Geometry: final body of the model. Coordinates: model frame, mm. A direction names the side the tool comes from. Give positions to 0.01 mm unless a question says otherwise; leave off trailing zeros. Loops run counter-clockwise (first coordinate to the right, second up) from the corner with the lowest first, then second, coordinate; pieces in that order, holes last. Notation, with made-up numbers: (63, 77.5) - (109, 77.5) arc R30 cw to (109, 100.5) - close; hole circle Ø5 at (-5.75, -15). An arc over 180 degrees is marked (long way). Use one line per item in the form item = value.
Autodesk Fusion 360 part; units mm, degrees
sketch "Sketch2" plane through (0, 0, 0) normal (0, 0, 1) x (1, 0, 0)
  line L0 (0, 0) -> (147.5, 0)
  line L1 (147.5, 0) -> (147.5, 58.5)
  line L2 (147.5, 58.5) -> (0, 58.5)
  line L3 (0, 58.5) -> (0, 0)
  line L4 (69.75, 0) -> (77.75, 0)
  line L5 (77.75, 0) -> (77.75, -8)
  line L6 (77.75, -8) -> (69.75, -8)
  line L7 (69.75, -8) -> (69.75, 0)
  line L8 (147.5, 24.75) -> (147.5, 32.75)
  line L9 (147.5, 32.75) -> (155.5, 32.75)
  line L10 (155.5, 32.75) -> (155.5, 24.75)
  line L11 (155.5, 24.75) -> (147.5, 24.75)
  line L12 (73.75, 58.5) -> (73.75, 0) construction
  line L13 (147.5, 28.75) -> (155.5, 28.75) construction
  line L14 (151.5, 32.75) -> (151.5, 24.75) construction
  circle A0 centre (151.5, 28.75) radius 1.875
  line L15 (-8, 24.75) -> (0, 24.75)
  line L16 (-8, 32.75) -> (-8, 24.75)
  line L17 (0, 32.75) -> (-8, 32.75)
  circle A1 centre (-4, 28.75) radius 1.875
  line L18 (69.75, -4) -> (77.75, -4) construction
  line L19 (73.75, 0) -> (73.75, -8) construction
  circle A2 centre (73.75, -4) radius 1.875
  point P0 (73.75, 0)
  point P1 (147.5, 28.75)
  point P2 (-8, 28.75)
  dimension "d8" = 147.5
  dimension "d9" = 58.5
  dimension "d12" = 8
  dimension "d13" = 8
  dimension "d14" = 8
  dimension "d15" = 8
  dimension "d16" = 8
  dimension "d17" = 3.75
  dimension "d18" = 3.75
extrude "Extrude1" add sketch "Sketch2" along normal blind 3
fillet "Fillet1" radius 1.5 12 edges at (77.75, 0, 1.5) (77.75, -8, 1.5) (69.75, -8, 1.5) (69.75, 0, 1.5) (0, 24.75, 1.5) (-8, 24.75, 1.5) (-8, 32.75, 1.5) (0, 32.75, 1.5) (155.5, 32.75, 1.5) (147.5, 32.75, 1.5) (147.5, 24.75, 1.5) (155.5, 24.75, 1.5)
sketch "Sketch3" plane through (0, 0, 3) normal (0, 0, 1) x (-1, 0, 0)
  arc A0 (-154, -24.75) -> (-155.5, -26.25) centre (-154, -26.25) ccw
  line L0 (-155.5, -26.25) -> (-155.5, -31.25)
  arc A1 (-155.5, -31.25) -> (-154, -32.75) centre (-154, -31.25) ccw
  line L1 (-154, -32.75) -> (-149, -32.75)
  arc A2 (-147.5, -34.25) -> (-149, -32.75) centre (-149, -34.25) ccw
  line L2 (-147.5, -34.25) -> (-147.5, -58.5)
  line L3 (-147.5, -58.5) -> (0, -58.5)
  line L4 (0, -58.5) -> (0, -34.25)
  arc A3 (1.5, -32.75) -> (0, -34.25) centre (1.5, -34.25) ccw
  line L5 (1.5, -32.75) -> (6.5, -32.75)
  arc A4 (6.5, -32.75) -> (8, -31.25) centre (6.5, -31.25) ccw
  line L6 (8, -31.25) -> (8, -26.25)
  arc A5 (8, -26.25) -> (6.5, -24.75) centre (6.5, -26.25) ccw
  line L7 (6.5, -24.75) -> (1.5, -24.75)
  arc A6 (0, -23.25) -> (1.5, -24.75) centre (1.5, -23.25) ccw
  line L8 (0, -23.25) -> (0, 0)
  line L9 (0, 0) -> (-68.25, 0)
  arc A7 (-69.75, 1.5) -> (-68.25, 0) centre (-68.25, 1.5) ccw
  line L10 (-69.75, 1.5) -> (-69.75, 6.5)
  arc A8 (-69.75, 6.5) -> (-71.25, 8) centre (-71.25, 6.5) ccw
  line L11 (-71.25, 8) -> (-76.25, 8)
  arc A9 (-76.25, 8) -> (-77.75, 6.5) centre (-76.25, 6.5) ccw
  line L12 (-77.75, 6.5) -> (-77.75, 1.5)
  arc A10 (-79.25, 0) -> (-77.75, 1.5) centre (-79.25, 1.5) ccw
  line L13 (-79.25, 0) -> (-147.5, 0)
  line L14 (-147.5, 0) -> (-147.5, -23.25)
  arc A11 (-149, -24.75) -> (-147.5, -23.25) centre (-149, -23.25) ccw
  line L15 (-149, -24.75) -> (-154, -24.75)
  circle A12 centre (-151.5, -28.75) radius 1.875
  circle A13 centre (4, -28.75) radius 1.875
  circle A14 centre (-73.75, 4) radius 1.875
  line L16 (0, -2.5) -> (-147.5, -2.5) construction
  line L17 (-54.6806, -2.5) -> (-92.6806, -2.5)
  line L18 (-92.6806, -2.5) -> (-92.6806, 0)
  line L19 (-54.6806, -2.5) -> (-54.6806, 0)
  line L20 (-54.6806, 0) -> (-92.6806, 0)
  line L21 (-145, -57) -> (-145, 0) construction
  line L22 (-145, -13.4089) -> (-145, -43.4089)
  line L23 (-145, -43.4089) -> (-147.5, -43.4089)
  line L24 (-145, -13.4089) -> (-147.5, -13.4089)
  line L25 (-147.5, -13.4089) -> (-147.5, -43.4089)
  line L26 (-73.75, -58.5) -> (-73.6806, 0) construction
  line L27 (-2.3933, -13.578) -> (0.1067, -13.5839)
  line L28 (0.1067, -13.5839) -> (0.0356, -43.5838)
  line L29 (-2.4644, -43.5779) -> (0.0356, -43.5838)
  line L30 (-2.3933, -13.578) -> (-2.4644, -43.5779)
  line L31 (0, -56) -> (-147.5, -56) construction
  line L32 (-50.7607, -56.0267) -> (-95.7606, -55.9733)
  line L33 (-95.7606, -55.9733) -> (-95.7606, -58.5)
  line L34 (-50.7607, -56.0267) -> (-50.7607, -58.5)
  line L35 (-50.7607, -58.5) -> (-95.7606, -58.5)
  line L36 (-70.7606, -56.003) -> (-75.7606, -55.997)
  line L37 (-75.7606, -55.997) -> (-75.7611, -58.5)
  line L38 (-75.7611, -58.5) -> (-70.7611, -58.5)
  line L39 (-70.7611, -58.5) -> (-70.7606, -56.003)
  point P0 (-73.6806, -2.5)
  point P1 (-145, -28.4089)
  point P2 (-73.2606, -56)
  point P3 (-73.2606, -56)
  dimension "d23" = 2.5
  dimension "d24" = 38
  dimension "d25" = 2.5
  dimension "d26" = 30
  dimension "d27" = 2.5
  dimension "d28" = 45
  dimension "d29" = 5
extrude "Extrude2" add sketch "Sketch3" along normal blind 15 contours L2 L14 L22 L23 L24 L25 | L9 L13 L17 L18 L19 L20 | L3 L32 L33 L35 L37 | L3 L32 L34 L35 L39 | A6 L8 L27 L28 | L4 A3 A6 L8 L27 L28 L29 L30 | L4 A3 L28 L29
equation "controller_length = 144 mm"
equation "controller_width = 55 mm"
equation "mount_hole_diameter = 3.5 mm"
equation "base_thickness = 3 mm"
equation "wall_thickness = 2.5 mm"
equation "give = 1 mm"
equation "d8 = total_length"
equation "d9 = total_width"
equation "total_length = controller_length + wall_thickness + give"
equation "total_width = controller_width + give + wall_thickness"
equation "d19 = base_thickness"
equation "d23 = wall_thickness"
equation "d25 = wall_thickness"
equation "d27 = wall_thickness"
equation "d30 = wall_height"
equation "wall_height = 15 mm"
(1) Cut plane B-B (y = -4). Return the cut outline in (x, z) (3 decimals), plus the area to 4 significant figures.
Solution:
outline = (69.75, 0) - (71.875, 0) - (71.875, 3) - (69.75, 3) - close; (75.625, 0) - (77.75, 0) - (77.75, 3) - (75.625, 3) - close
area = 12.75 mm2
(2) Access query for faces 1 (the face through (149.7, 27.6, 3)), 2 (the face through (151, 32.75, 1)), 3 (the face through (73, 2.5, 10)). Directions: +Z, -Z, +X, -X, +Y, -Y. A direction counts if a zero-diameter tool reaches every point of the face in a straight line with its end or side. Return the directions, or none.
Solution:
face_1 = +Z, +X, +Y, -Y
face_2 = +Z, -Z, +X, +Y
face_3 = +Z, +X, -X
(3) Cut plane A-A (z = 16). Return the cut outline in (x, y), plus the area to 3 significant figures.
Solution:
outline = (-0.11, 13.58) - (2.39, 13.58) - (2.46, 43.58) - (-0.04, 43.58) - close; (50.76, 56.03) - (70.76, 56) - (70.76, 58.5) - (50.76, 58.5) - close; (54.68, 0) - (92.68, 0) - (92.68, 2.5) - (54.68, 2.5) - close; (75.76, 56) - (95.76, 55.97) - (95.76, 58.5) - (75.76, 58.5) - close; (145, 13.41) - (147.5, 13.41) - (147.5, 43.41) - (145, 43.41) - close
area = 345 mm2
(4) Pull-direction query (Y, two-part tool) for faces 4 (the face through (-4.41, 30.58, 1.48)), 5 (the face through (0, 12, 1)), 6 (the face through (73, 0, 7)), 7 (the face through (72.4, -5.3, 1.5)); classes: released by +Y, released by -Y, zero draft, split by the parting line, or undercut.
Solution:
face_4 = undercut
face_5 = zero draft
face_6 = released by -Y
face_7 = undercut
(5) Cut plane D-D (x = 73.75). Return the cut outline in (y, z) (3 decimals).
Solution:
outline = (-8, 0) - (-5.875, 0) - (-5.875, 3) - (-8, 3) - close; (-2.125, 0) - (58.5, 0) - (58.5, 3) - (2.5, 3) - (2.5, 18) - (0, 18) - (0, 3) - (-2.125, 3) - close
(6) Material intervals for L1, parallel to X at y = 37, z = 16.75; L2, parallel to Y at x = 87, z = 16.75; L3, parallel to Y at x = 73.75, z = 0.9 (3 decimals), sorted ascending. Write a range as from..to.
Solution:
L1 = -0.05..2.45, 145..147.5
L2 = 0..2.5, 55.98..58.5
L3 = -8..-5.875, -2.125..58.5
(7) Pin query (flat end, axial travel): P1, Ø1.5, axis at y = -3.5, z = 1, coming from the +X side; P2, Ø0.9, axis at y = 51.5, z = 2, coming from the -X side; P3, Ø4, axis at x = 74.5, y = -5.5, coming from the +Z side; P4, Ø3.5, axis at x = 73.75, y = -4, coming from the -Z side. Return the tip coordinate at first contact, or that it passes through.
Solution:
P1 = 77.75
P2 = 0
P3 = 3
P4 = through
(8) Cut plane C-C (x = -4). Return the cut outline in (y, z) (3 decimals), plus the area to 4 significant figures.
Solution:
outline = (24.75, 0) - (26.875, 0) - (26.875, 3) - (24.75, 3) - close; (30.625, 0) - (32.75, 0) - (32.75, 3) - (30.625, 3) - close
area = 12.75 mm2
